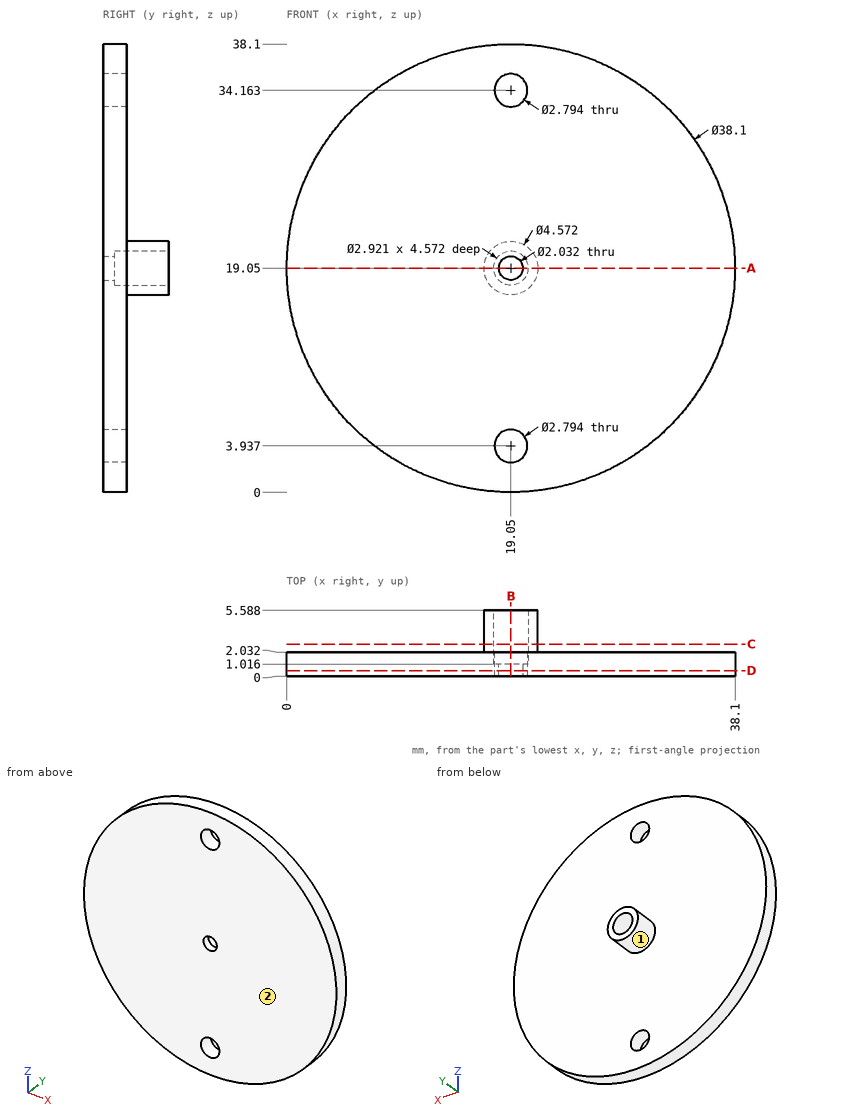
Study the drawing (mm; zero at the part's minimum x, y, z) and answer. A direction names the side the tool comes from. Coordinates: 2 decimals unless noted, no trailing zeros. Loops run counter-clockwise (first coordinate to the right, second up) from the corner with the lowest first, then second, coordinate; pieces in that order, holes last. Notation, with made-up numbers: M 55.25,70 L 91.25,70 A21 ccw 91.25,102 Z; hole C 24,57 d6. An arc over 180 degrees is marked long. Answer in a Markdown table with one row per item.
1) Find section C-C (y = 2.7). Determine the outline of the cut face in (x, z).
Answers below:
| item | result |
|---|---|
| outline | C 19.05,19.05 d4.57; hole C 19.05,19.05 d2.92 |
2) Find section D-D (y = 0.45). Determine the outline of the cut face in (x, z).
Answers below:
| item | result |
|---|---|
| outline | C 19.05,19.05 d38.1; hole C 19.05,3.94 d2.79; hole C 19.05,34.16 d2.79; hole C 19.05,19.05 d2.03 |
3) Which of the six approach directions +Z, -Z, +X, -X, +Y, -Y give full straight-line access (tool end or side, diameter ignored) to the marked faces 1 and 2?
Answers below:
| item | result |
|---|---|
| face 1 | +Y |
| face 2 | +Z, -Z, +X, -X, -Y |
4) Find section A-A (z = 19.05). Determine the outline of the cut face in (x, y).
Answers below:
| item | result |
|---|---|
| outline | M 0,0 L 18.03,0 L 18.03,1.02 L 17.59,1.02 L 17.59,5.59 L 16.76,5.59 L 16.76,2.03 L 0,2.03 Z; M 20.07,0 L 38.1,0 L 38.1,2.03 L 21.34,2.03 L 21.34,5.59 L 20.51,5.59 L 20.51,1.02 L 20.07,1.02 Z |
5) Given pin 1 (1.6 mm diameter, centred on x = 19.05, z = 19.05, fed in from -Y); pin 2 (2.5 mm diameter, centred on x = 19, z = 19, fed in from +Y), each flat-ended and moving along its own axis, determine where each tip first touches the part or whether it passes through.
Answers below:
| item | result |
|---|---|
| pin 1 | through |
| pin 2 | y = 1.02 |
6) Find section B-B (x = 19.05). Determine the outline of the cut face in (y, z).
Answers below:
| item | result |
|---|---|
| outline | M 0,0 L 2.03,0 L 2.03,2.54 L 0,2.54 Z; M 0,5.33 L 2.03,5.33 L 2.03,16.76 L 5.59,16.76 L 5.59,17.59 L 1.02,17.59 L 1.02,18.03 L 0,18.03 Z; M 0,20.07 L 1.02,20.07 L 1.02,20.51 L 5.59,20.51 L 5.59,21.34 L 2.03,21.34 L 2.03,32.77 L 0,32.77 Z; M 0,35.56 L 2.03,35.56 L 2.03,38.1 L 0,38.1 Z |
7) Find the intervals of material crossed by probe 1 along Z at (x, y) = (19.05, 0.75); probe 2 along Z at (x, y) = (19.05, 2.5), in increasing order.
Answers below:
| item | result |
|---|---|
| probe 1 | 0 to 2.54, 5.33 to 18.03, 20.07 to 32.77, 35.56 to 38.1 |
| probe 2 | 16.76 to 17.59, 20.51 to 21.34 |
